Build history of the part. All positions in model axes, mm. Face numbers are marked on the shaded views. A direction names the side the tool comes from. Give positions to 0.01 mm unless a question says otherwise; leave off trailing zeros. Order: outer loops, then holes, each group sorted by start corner. A loop starts at its lowest first (then second) coordinate and runs counter-clockwise, first axis right, second up. Notation, with made-up numbers: M 47,-20 L 58,-20 A23 cw 58,-11 Z; hole C 69,82 d4. An arc over 180 degrees is marked long. One line per item, written item: value.
from build123d import *

# Parameters (mm, degrees)
BASEHEAD_DEPTH     = 3.65
INDENT_START       = -0.45625
INDENT_2_OUTLINE_R = 3.5
INDENT_2_DEPTH     = 0.45625
SKETCH4_W          = 0.5
SKETCH4_H          = 10.618802154
THDSCHPAT_COUNT    = 8
THDSCHPAT_PITCH    = 0.775


# Read off the part's stored shape, not the designer's step: Indent
with BuildPart() as part:
    # Sketch1 → BaseHead (new body)
    with BuildSketch(Plane(origin=(0, 0, 0), x_dir=(0, 0, -1), z_dir=(1, 0, 0))):
        Polygon((4, 2.309401077), (4, -2.309401077), (0, -4.618802154), (-4, -2.309401077), (-4, 2.309401077), (0, 4.618802154), align=None)
    extrude(amount=BASEHEAD_DEPTH)

    # Indent outline → Indent (revolve)
    with BuildSketch(Plane.YX):
        Polygon((2.5, 3.65), (2.5, 14.405), (2.055, 14.85), (0, 14.85), (0, 3.65), align=None)
    revolve(axis=Axis((0, 0, 0), (1, 0, 0)))

    # Indent 2 outline → Indent 2 (cut)
    with BuildSketch(Plane.ZY.offset(INDENT_START)):
        with Locations((0.033212245, 0.192376607)):
            Circle(INDENT_2_OUTLINE_R)
    extrude(amount=INDENT_2_DEPTH, mode=Mode.SUBTRACT)

    # Sketch3 → HeadChamfer (revolve, cut)
    with BuildSketch(Plane.XY, mode=Mode.PRIVATE) as headchamfer_sk:
        Polygon((0, 4), (3.244016936, 9.618802154), (3.244016936, 14.618802154), (-10, 14.618802154), (-10, 4), align=None)
    revolve(headchamfer_sk.sketch.rotate(Axis((0, 0, 0), (1, 0, 0)), 90), axis=Axis((0, 0, 0), (1, 0, 0)), mode=Mode.SUBTRACT)

    # Sketch4 → BearingFace (revolve, cut)
    with BuildSketch(Plane.XY, mode=Mode.PRIVATE) as bearingface_sk:
        with Locations((3.4, 9.309401077)):
            Rectangle(SKETCH4_W, SKETCH4_H)
    revolve(bearingface_sk.sketch.rotate(Axis((0, 0, 0), (1, 0, 0)), 90), axis=Axis((0, 0, 0), (1, 0, 0)), mode=Mode.SUBTRACT)

    # ThdSchSke → ThreadSchematic (revolve, cut)
    with BuildSketch(Plane.XY):
        Polygon((8.65, -2.055), (8.338407645, -2.5), (8.338407645, -3.125), (8.961592355, -3.125), (8.961592355, -2.5), align=None)
    threadschematic = revolve(axis=Axis((-3.175, 0, 0), (1, 0, 0)), mode=Mode.SUBTRACT)

    # ThdSchPat: ThreadSchematic ×8
    with Locations(*[(i * THDSCHPAT_PITCH, 0, 0) for i in range(1, THDSCHPAT_COUNT)]):
        add(threadschematic, mode=Mode.SUBTRACT)


solid = part.part
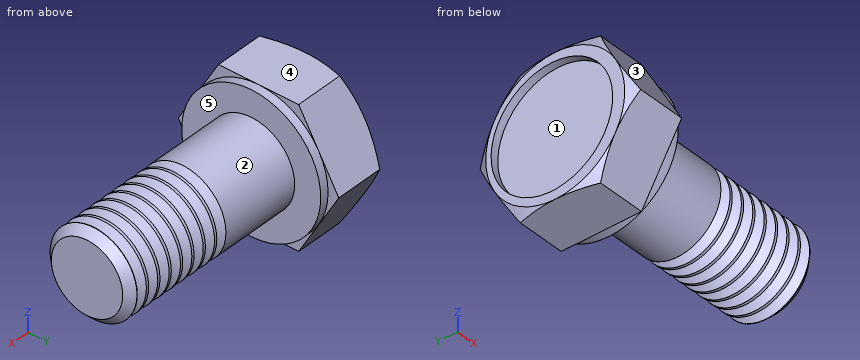
1) Tool access for the marked faces 4 and 5: list every direction of +Z, -Z, +X, -X, +Y, -Y with a clear straight run to the whole face (end or side of a thin tool).
Check values:
face 4: +Z, +X, -X, +Y, -Y
face 5: +X
2) Pin check, flat tips, straight feed: pin 1 (1 mm diameter, centred on y = -2, z = 3, fed in from +X); pin 2 (1.6 mm diameter, centred on y = 2, z = 2.5, fed in from +X); pin 3 (1 mm diameter, centred on x = 9, y = 3.5, fed in from +Z); pin 4 (1 mm diameter, centred on x = 4.5, z = 0, fed in from -Y). Stop position of each tip, or through.
Check values:
pin 1: x = 3.65
pin 2: x = 14.5
pin 3: through
pin 4: y = -2.5
3) Saw through at B-B, the plane x = 6. Write the cut outline in (y, z).
Check values:
outline: C 0,0 d5
4) Saw through at A-A, the plane x = 1.5. Write the cut outline in (y, z).
Check values:
outline: M -4.62,0 L -2.31,-4 L 2.31,-4 L 4.62,0 L 2.31,4 L -2.31,4 Z
5) Mould opens along Z. For the marked faces 1, 2 and 3 say: released by +Z, released by -Z, zero draft, split by the parting line, or undercut.
Check values:
face 1: undercut
face 2: split by the parting line
face 3: released by +Z
6) Drill centre lines: probe 1 along Y at (x, z) = (9, 0); probe 2 along Z at (x, y) = (5.25, 1.5); probe 3 along X at (y, z) = (-1.5, 0.75). Where is each one in solid material? Low to high. Write a range as from..to.
Check values:
probe 1: -2.5..2.5
probe 2: -2..2
probe 3: 0.46..14.85
